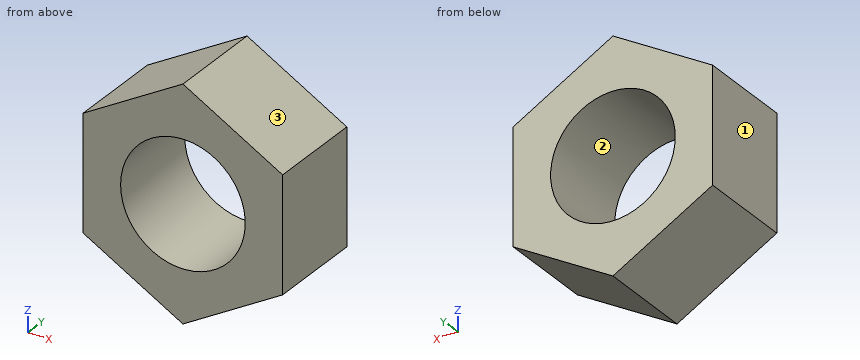
Autodesk Inventor part; units mm, degrees
ref_plane "YZ Plane" through (0, 0, 0) normal (1, 0, 0) x (0, 1, 0)
ref_plane "XZ Plane" through (0, 0, 0) normal (0, 1, 0) x (-1, 0, 0)
ref_plane "XY Plane" through (0, 0, 0) normal (0, 0, 1) x (1, 0, 0)
sketch "Skizze3" plane through (0, 0, 0) normal (0, 1, 0) x (-1, 0, 0)
  circle A0 centre (0, 0) radius 2.5
  line L0 (4, 0) -> (4, 9.599)
  line L1 (4, 9.599) -> (4, -8.7779)
  line L2 (-4, 0) -> (-4, 9.2876)
  line L3 (-4, 9.2876) -> (-4, -8.3814)
  line L4 (-6.313, 8.2636) -> (9.6019, -0.9248)
  line L5 (-10.313, -1.3354) -> (5.6019, 7.853)
  line L6 (-4, -9.599) -> (-4, 8.7779)
  line L7 (6.313, -8.2636) -> (-9.6019, 0.9248)
  line L8 (10.313, 1.3354) -> (-5.6019, -7.853)
  point P0 (0, -4.6188)
  point P1 (4, -2.3094)
  point P2 (4, 2.3094)
  point P3 (0, 4.6188)
  point P4 (-4, 2.3094)
  point P5 (-4, -2.3094)
  dimension "d34" = 5
  dimension "d38" = 360
extrude "Extrusion1" add sketch "Skizze3" along normal blind 4 contours L1 L8 L7 L3 L2 L5 L4 L0
properties part number "01-03-01 Kugellager" material "Stahl, Guss"
Can you work these out from the model? Positions are in its coordinate system, mm. Face numbers are marked on the shaded views. Round coordinates to 2 decimals unless told otherwise and drop trailing zeros. Loops run counter-clockwise (first coordinate to the right, second up) from the corner with the lowest first, then second, coordinate; pieces in that order, holes last. Notation, with made-up numbers: M 49.5,48 L 104.5,48 A31 ccw 104.5,83 Z; hole C -17.5,-38.5 d7. An arc over 180 degrees is marked long. Write item = value, one per line. Start each with the question number.
(1) Suppose I cut it at B-B on y = 1.4. Write out the boundary of the cut face in (x, z).
(2) I need wall thicknesses on line 1 along Z through (x, y) = (1, 3.05); line 2 along Z through (x, y) = (-1.75, 2.45); line 3 along Z through (x, y) = (2.75, 0.6). Which ranges of each line are inside material? Lowest first, please.
(3) I'm going to push a flat-ended pin straight in: P1, Ø1.5, axis at x = -0.5, y = 1.5, coming from the -Z side. Where does the tip first touch, or does it pass through?
(4) Suppose I cut it at A-A on z = 0. Write out the boundary of the cut face in (x, y), plus the area to 3 significant figures.
(5) If we mould it in two halves opening along Z, with no side actions, what happens to the marked faces 1, 2 and 3? For each: released by +Z, released by -Z, zero draft, split by the parting line, or undercut.
(6) Suppose I cut it at C-C on x = 0.75. Write out the boundary of the cut face in (y, z), plus the area to 3 significant figures.
Answer block:
q1.outline = M -4,-2.31 L 0,-4.62 L 4,-2.31 L 4,2.31 L 0,4.62 L -4,2.31 Z; hole C 0,0 d5
q2.line_1 = -4.04 to -2.29, 2.29 to 4.04
q2.line_2 = -3.61 to -1.79, 1.79 to 3.61
q2.line_3 = -3.03 to 3.03
q3.P1 = -4.62
q4.outline = M -4,0 L -2.5,0 L -2.5,4 L -4,4 Z; M 2.5,0 L 4,0 L 4,4 L 2.5,4 Z
q4.area = 12.0 mm²
q5.face_1 = zero draft
q5.face_2 = undercut
q5.face_3 = released by +Z
q6.outline = M 0,-4.19 L 4,-4.19 L 4,-2.38 L 0,-2.38 Z; M 0,2.38 L 4,2.38 L 4,4.19 L 0,4.19 Z
q6.area = 14.4 mm²
